Print and shaded views of the part. All mm, measured from the part's lowest x, y and z. A direction names the side the tool comes from. Coordinates: 2 decimals unless noted, no trailing zeros. Order: outer loops, then holes, each group sorted by start corner. A loop starts at its lowest first (then second) coordinate and runs counter-clockwise, first axis right, second up. Notation, with made-up numbers: (-9.5, -39.75) -> (6.5, -39.75) arc R25 cw to (6.5, -2.75) -> close; hole circle Ø4 at (42.25, 32). An arc over 180 degrees is marked (long way). Use one line per item in the form item = value. Start each with the question number.
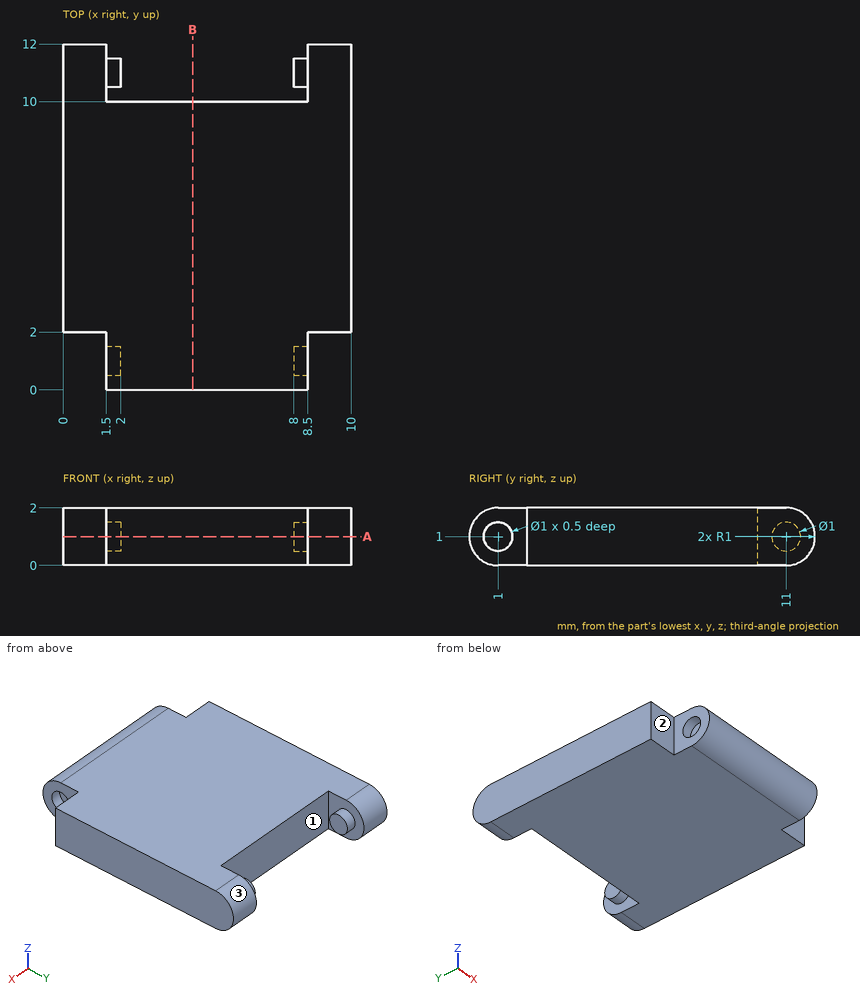
1) 3-axis set-ups, long thin cutter, end or side, ignore diameter. For the marked faces 1, 2 and 3: which of +Z, -Z, +X, -X, +Y, -Y reach the whole face in a straight line?
2) Drop flat-ended pins along their axis: P1, Ø0.8, axis at x = 0.5, z = 0.5, coming from the -Y side; P2, Ø1, axis at x = 5, z = 1.5, coming from the +Y side; P3, Ø0.6, axis at y = 0.5, z = 1.5, coming from the -X side; P4, Ø1.1, axis at y = 11, z = 1, coming from the -X side. Give the stop position or say it passes through.
3) Cut at B-B on x = 4.5. Give the cut face in (y, z).
4) Cut at A-A on z = 1. Give the cut face in (x, y).
5) Probe L1, parallel to Z at x = 1.8, y = 1; L2, parallel to X at y = 10.25, z = 1; L3, parallel to Y at x = 3.75, z = 1. List the from-to ranges inside material, lowest first.
Values follow:
q1.face_1 = +Z, -Z
q1.face_2 = +Z, -Z, -X, -Y
q1.face_3 = +X, -X, +Y
q2.P1 = 2
q2.P2 = 10
q2.P3 = 1.5
q2.P4 = 0
q3.outline = (1, 0) -> (10, 0) -> (10, 2) -> (1, 2) arc R1 ccw to start
q4.outline = (0, 2) -> (1.5, 2) -> (1.5, 1.5) -> (2, 1.5) -> (2, 0.5) -> (1.5, 0.5) -> (1.5, 0) -> (8.5, 0) -> (8.5, 0.5) -> (8, 0.5) -> (8, 1.5) -> (8.5, 1.5) -> (8.5, 2) -> (10, 2) -> (10, 12) -> (8.5, 12) -> (8.5, 11.5) -> (8, 11.5) -> (8, 10.5) -> (8.5, 10.5) -> (8.5, 10) -> (1.5, 10) -> (1.5, 10.5) -> (2, 10.5) -> (2, 11.5) -> (1.5, 11.5) -> (1.5, 12) -> (0, 12) -> close
q5.L1 = 0 to 0.5, 1.5 to 2
q5.L2 = 0 to 1.5, 8.5 to 10
q5.L3 = 0 to 10
